Build history of the part. All positions in model axes, mm. Coordinates: 2 decimals unless noted, no trailing zeros. Loops run counter-clockwise (first coordinate to the right, second up) from the corner with the lowest first, then second, coordinate; pieces in that order, holes last. Notation, with made-up numbers: (35.5, -17.5) - (74.5, -17.5) arc R21 cw to (74.5, 13.5) - close; hole circle Ø11 at (39, 12.25). An arc over 180 degrees is marked (long way). One line per item, written item: value.
```python
from build123d import *

# Parameters (mm, degrees)
BOSS_EXTRUDE1_DEPTH = 0.3
SKETCH2_R           = 0.6
CUT_EXTRUDE2_DEPTH  = 0.3
CUT_EXTRUDE3_DEPTH  = 0.1


with BuildPart() as part:
    # Sketch1 → Boss-Extrude1 (new body)
    with BuildSketch(Plane(origin=(0, 0, 0), x_dir=(1, 0, 0), z_dir=(0, 1, 0))):
        with BuildLine():
            Line((-0.268357858, 1.770915819), (-0.268357858, 0.8908721))
            ThreePointArc((-0.268357858, 0.8908721), (0, -0.93041337), (0.268357858, 0.8908721))
            Line((0.268357858, 0.8908721), (0.268357858, 1.770915819))
            Line((0.268357858, 1.770915819), (0.380994594, 1.770915819))
            Line((0.380994594, 1.770915819), (0.6, 8.4))
            Line((0.6, 8.4), (0, 9))
            Line((0, 9), (-0.6, 8.4))
            Line((-0.6, 8.4), (-0.380994594, 1.770915819))
            Line((-0.380994594, 1.770915819), (-0.268357858, 1.770915819))
        make_face()
    extrude(amount=BOSS_EXTRUDE1_DEPTH)

    # Sketch2 → Cut-Extrude2 (cut)
    with BuildSketch(Plane(origin=(0, 0, 0), x_dir=(1, 0, 0), z_dir=(0, 1, 0))):
        Circle(SKETCH2_R)
    extrude(amount=CUT_EXTRUDE2_DEPTH, mode=Mode.SUBTRACT)

    # Sketch4 → Cut-Extrude3 (cut)
    with BuildSketch(Plane(origin=(0, 0.3, 0), x_dir=(1, 0, 0), z_dir=(0, 1, 0))):
        Polygon((0, 8.662563121), (0.377183269, 8.285379851), (0.188591635, 2.014863516), (-0.188591635, 2.014863516), (-0.377183269, 8.285379851), align=None)
    extrude(amount=-CUT_EXTRUDE3_DEPTH, mode=Mode.SUBTRACT)


solid = part.part
```
Item 1: Cut at B-B, the plane z = -0.5. Write the cut outline in (x, y).
Check result:
outline: (-0.78, 0) - (-0.33, 0) - (-0.33, 0.3) - (-0.78, 0.3) - close; (0.33, 0) - (0.78, 0) - (0.78, 0.3) - (0.33, 0.3) - close
Item 2: Cut at D-D, the plane z = -1.5. Write the cut outline in (x, y).
Check result:
outline: (-0.27, 0) - (0.27, 0) - (0.27, 0.3) - (-0.27, 0.3) - close
Item 3: Cut at C-C, the plane z = -6. Write the cut outline in (x, y).
Check result:
outline: (-0.52, 0) - (0.52, 0) - (0.52, 0.3) - (0.31, 0.3) - (0.31, 0.2) - (-0.31, 0.2) - (-0.31, 0.3) - (-0.52, 0.3) - close
Item 4: Probe probe 1 along X at (y, z) = (0.25, 0); probe 2 along X at (y, z) = (0.1, -1.25); probe 3 along Y at (x, z) = (-0.1, -5.25). List the from-to ranges inside material, lowest first. Write a range as from..to.
Check result:
probe 1: x = -0.93..-0.6, 0.6..0.93
probe 2: x = -0.27..0.27
probe 3: y = 0..0.2
Item 5: Cut at A-A, the plane y = 0.1. Write the cut outline in (x, z).
Check result:
outline: (-0.6, -8.4) - (0, -9) - (0.6, -8.4) - (0.38, -1.77) - (0.27, -1.77) - (0.27, -0.89) arc R0.93 ccw (long way) to (-0.27, -0.89) - (-0.27, -1.77) - (-0.38, -1.77) - close; hole circle Ø1.2 at (0, 0)
Item 6: Drop a flat-ended pin along its axis: P1, Ø0.7, axis at x = 0, z = 0, coming from the +Y side. Give the stop position or say it passes through.
Check result:
P1: passes through
